Verification items for the finished model (mm, model axes). Face numbers are marked on the shaded views. A direction names the side the tool comes from. Give positions to 0.01 mm unless a question says otherwise; leave off trailing zeros. Order: outer loops, then holes, each group sorted by start corner. A loop starts at its lowest first (then second) coordinate and runs counter-clockwise, first axis right, second up.
(1) Mould release check, pull along Y, two halves, no side actions. Record for the marked faces 4, 5 and 6: pulls with the +Y half, pulls with the -Y half, needs draft (parallel to the pull), parting line crosses it, or undercut.
(2) Gauge pin test, flat end, axial feed: pin 1 (6 mm diameter, centred on x = 43, z = -15, fed in from +Y). Record the tip position at first contact, or that the pin passes through.
(3) Sectioned sample at B-B on z = -13. Record the cut outline in (x, y), plus the area to 3 significant figures.
(4) Sectioned sample at D-D on y = 15.75. Record the cut outline in (x, z).
(5) Sectioned sample at C-C on x = 33. Record the cut outline in (y, z).
(6) Sectioned sample at A-A on y = 10. Record the cut outline in (x, z).
(7) Scan lines: L1, parallel to X at y = 2.75, z = -5.25; L2, parallel to X at y = 11, z = -16.75; L3, parallel to Z at x = 10, y = 3.75. Record each from-to range of solid material in increasing order.
(8) Access from +Z, -Z, +X, -X, +Y, -Y to the whole of each face (thin tool, end or side, straight path). Record for the marked faces 1, 2 and 3.
```python
from build123d import *

# Parameters (mm, degrees)
SKETCH1_W                = 51.3
SKETCH1_H                = 27.6
SKETCH1_W_2              = 47.3
SKETCH1_H_2              = 23.6
EXTRUDE_THIN1_DEPTH      = 17
SKETCH2_W                = 51.3
SKETCH2_H                = 27.6
BOSS_EXTRUDE1_DEPTH      = 1.2
SKETCH3_W                = 30.5
SKETCH3_H                = 14.5
CUT_EXTRUDE1_DEPTH       = 10
SKETCH7_W                = 7
SKETCH7_H                = 23.6
SKETCH7_W_2              = 5.65
BOSS_EXTRUDE2_DEPTH      = 3
BOSS_EXTRUDE3_DEPTH      = 15
BOSS_EXTRUDE3_DEPTH_BACK = 15
FILLET1_R                = 1
SKETCH12_W               = 9
SKETCH12_H               = 12
CUT_EXTRUDE3_DEPTH       = 10
SKETCH14_W               = 1.5
SKETCH14_H               = 3
BOSS_EXTRUDE4_DEPTH      = 4


with BuildPart() as part:
    # Sketch1 → Extrude-Thin1 (new body)
    with BuildSketch(Plane(origin=(0, 0, 0), x_dir=(1, 0, 0), z_dir=(0, 1, 0))):
        with Locations((23.65, 11.8)):
            Rectangle(SKETCH1_W, SKETCH1_H)
        with Locations((23.65, 11.8)):
            Rectangle(SKETCH1_W_2, SKETCH1_H_2, mode=Mode.SUBTRACT)
    extrude(amount=EXTRUDE_THIN1_DEPTH)

    # Sketch2 → Boss-Extrude1 (add)
    with BuildSketch(Plane.XZ):
        with Locations((23.65, -11.8)):
            Rectangle(SKETCH2_W, SKETCH2_H)
    extrude(amount=BOSS_EXTRUDE1_DEPTH)

    # Sketch3 → Cut-Extrude1 (cut)
    with BuildSketch(Plane(origin=(0, 0, 0), x_dir=(1, 0, 0), z_dir=(0, 1, 0))):
        with Locations((26.4, 11.8)):
            Rectangle(SKETCH3_W, SKETCH3_H)
    extrude(amount=-CUT_EXTRUDE1_DEPTH, mode=Mode.SUBTRACT)

    # Sketch7 → Boss-Extrude2 (add)
    with BuildSketch(Plane(origin=(0, 0, 0), x_dir=(1, 0, 0), z_dir=(0, 1, 0))):
        with Locations((3.5, 11.8)):
            Rectangle(SKETCH7_W, SKETCH7_H)
        with Locations((44.475, 11.8)):
            Rectangle(SKETCH7_W_2, SKETCH7_H)
    extrude(amount=BOSS_EXTRUDE2_DEPTH)

    # Sketch9 → Boss-Extrude3 (add, two sides)
    with BuildSketch(Plane.ZY.offset(-24)) as boss_extrude3_sk:
        Polygon((-22.6, 11), (-23.6, 12), (-23.6, 11), align=None)
        Polygon((0, 12), (-1, 11), (0, 11), align=None)
    extrude(amount=BOSS_EXTRUDE3_DEPTH)
    extrude(boss_extrude3_sk.sketch, amount=-BOSS_EXTRUDE3_DEPTH_BACK)

    # Fillet1
    fillet1_edges = [part.edges().sort_by_distance(p)[0] for p in [
        (-2, -1.2, -11.8),
        (23.65, -1.2, -25.6),
        (49.3, -1.2, -11.8),
        (23.65, -1.2, 2),
        (-2, 7.9, -25.6),
        (49.3, 7.9, -25.6),
        (49.3, 7.9, 2),
        (-2, 7.9, 2),
    ]]
    fillet(fillet1_edges, radius=FILLET1_R)

    # Sketch12 → Cut-Extrude3 (cut)
    with BuildSketch(Plane.ZY.offset(2)):
        with Locations((-11.8, 17)):
            Rectangle(SKETCH12_W, SKETCH12_H)
    extrude(amount=-CUT_EXTRUDE3_DEPTH, mode=Mode.SUBTRACT)

    # Sketch14 → Boss-Extrude4 (add)
    with BuildSketch(Plane(origin=(0, 4.8, 0), x_dir=(1, 0, 0), z_dir=(0, 1, 0))):
        with Locations((0.75, 22.1)):
            Rectangle(SKETCH14_W, SKETCH14_H)
        with Locations((46.55, 22.1)):
            Rectangle(SKETCH14_W, SKETCH14_H)
        with Locations((46.55, 1.5)):
            Rectangle(SKETCH14_W, SKETCH14_H)
        with Locations((0.75, 1.5)):
            Rectangle(SKETCH14_W, SKETCH14_H)
    extrude(amount=BOSS_EXTRUDE4_DEPTH)


solid = part.part
```
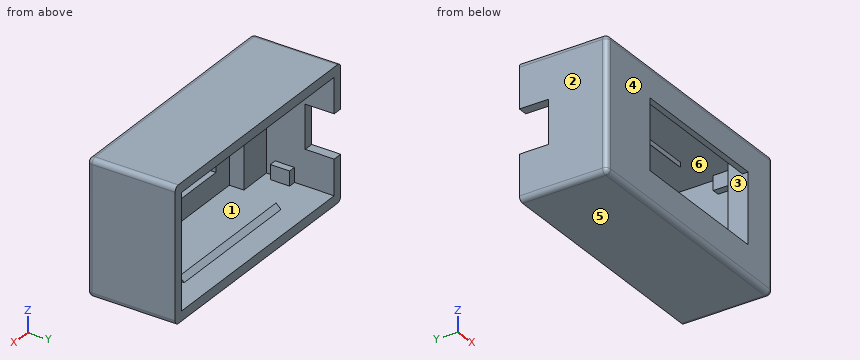
Ans:
1. face 4: pulls with the -Y half
1. face 5: needs draft
1. face 6: undercut
2. pin 1: stops at y = 3
3. outline: (-2, -0.2) arc R1 ccw to (-1, -1.2) - (11.15, -1.2) - (11.15, 0) - (7, 0) - (7, 3) - (0, 3) - (0, 11) - (-2, 11) - close; (41.65, -1.2) - (48.3, -1.2) arc R1 ccw to (49.3, -0.2) - (49.3, 17) - (47.3, 17) - (47.3, 3) - (41.65, 3) - close
3. area: 118 mm2
4. outline: (-2, -24.6) arc R1 ccw to (-1, -25.6) - (48.3, -25.6) arc R1 ccw to (49.3, -24.6) - (49.3, 1) arc R1 ccw to (48.3, 2) - (-1, 2) arc R1 ccw to (-2, 1) - (-2, -7.3) - (0, -7.3) - (0, 0) - (47.3, 0) - (47.3, -23.6) - (0, -23.6) - (0, -16.3) - (-2, -16.3) - close
5. outline: (-1.2, -24.6) arc R1 ccw to (-0.2, -25.6) - (17, -25.6) - (17, -23.6) - (12, -23.6) - (11, -22.6) - (11, -23.6) - (0, -23.6) - (0, -19.05) - (-1.2, -19.05) - close; (-1.2, -4.55) - (0, -4.55) - (0, 0) - (11, 0) - (11, -1) - (12, 0) - (17, 0) - (17, 2) - (-0.2, 2) arc R1 ccw to (-1.2, 1) - close
6. outline: (-2, -24.6) arc R1 ccw to (-1, -25.6) - (48.3, -25.6) arc R1 ccw to (49.3, -24.6) - (49.3, 1) arc R1 ccw to (48.3, 2) - (-1, 2) arc R1 ccw to (-2, 1) - close; hole (0, -23.6) - (47.3, -23.6) - (47.3, 0) - (0, 0) - close
7. L1: x = -2 to 7, 41.65 to 49.3
7. L2: x = -2 to 0, 47.3 to 49.3
7. L3: z = -25.6 to -23.6, 0 to 2
8. face 1: none
8. face 2: +Z, -Z, -X, +Y, -Y
8. face 3: +Y
